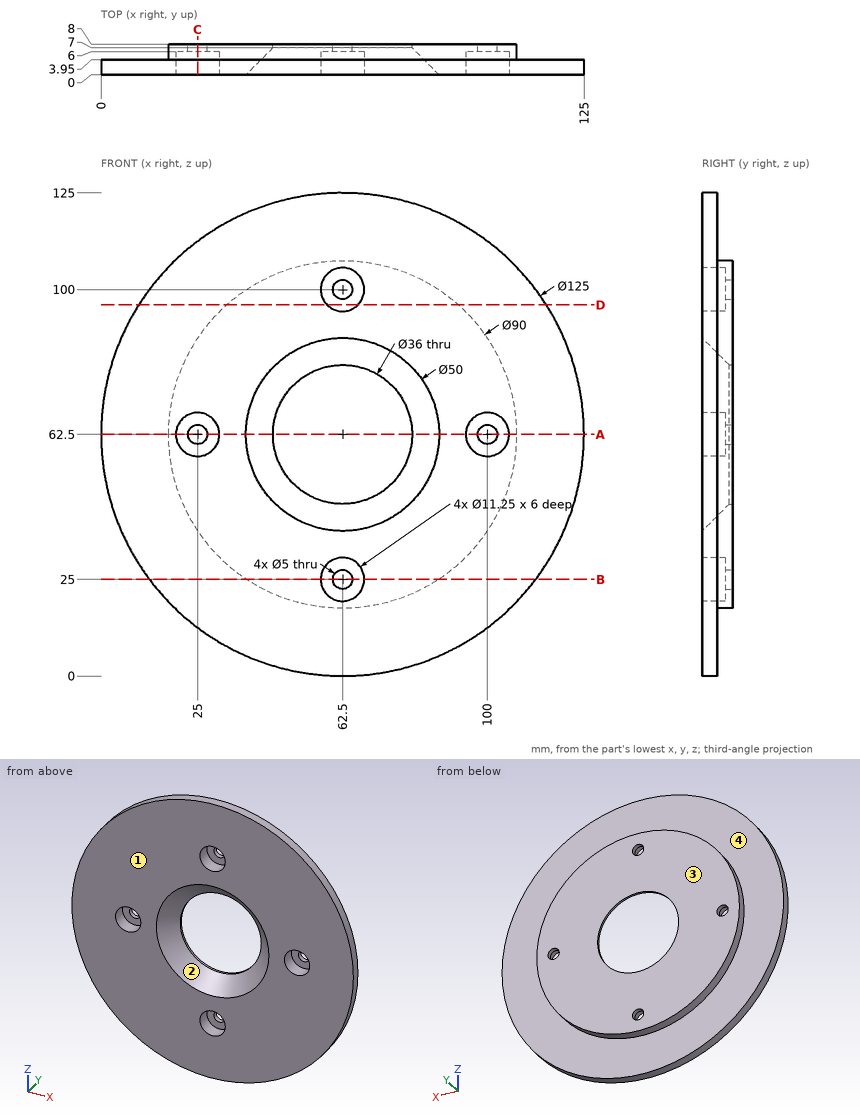
Source: three-view drawing plus pictorial views. Frame: mm from the lowest corner of the part. A direction names the side the tool comes from. Give positions to 0.01 mm unless a question says otherwise; leave off trailing zeros. Order: outer loops, then holes, each group sorted by start corner. A loop starts at its lowest first (then second) coordinate and runs counter-clockwise, first axis right, second up. Notation, with made-up numbers: (-22, -11.75) - (-16, -11.75) arc R23 cw to (-16, 17.25) - close; hole circle Ø6 at (14, -33). An arc over 180 degrees is marked (long way). Answer as a JSON object with one key per item and string values. Group by question number.
Q1. Line query: probe 1 along X at (y, z) = (3, 67.5); probe 2 along Z at (x, y) = (62.5, 7); probe 3 along Z at (x, y) = (62.5, 2.2) (3 decimals). Output: solid intervals per line, ascending.
Q2. Mould query, pull axis X, two halves, no side actions, for the marked faces 1 and 2. Classes: pulls with the +X half, pulls with the -X half, needs draft (parallel to the pull), parting line crosses it, or undercut.
Q3. First-contact query: pin 1 Ø3.5 at (x, z) = (61.5, 101.5) entering from -Y; pin 2 Ø2 at (y, z) = (3.5, 93) entering from +X; pin 3 Ø1 at (x, y) = (61, 1.5) entering from -Z. Flat tips, straight axial feed; report the tip coordinate or a pass-through.
Q4. Cut plane D-D, the plane z = 96. Output: boundary loops of the cut face in (x, y), then the cut area to 3 significant figures.
Q5. Cut plane C-C, the plane x = 25. Output: boundary loops of the cut face in (y, z) (3 decimals), then the cut area to 3 significant figures.
Q6. Cut plane B-B, the plane z = 25. Output: boundary loops of the cut face in (x, y) (3 decimals).
Q7. Set-up query: the marked faces 3 and 4. Return all of +Z, -Z, +X, -X, +Y, -Y with unobstructed straight access to the full face (end or side cutting, diameter ignored); none if empty.
Q8. Cut plane A-A, the plane z = 62.5. Count the separate pieces of the cut face and the enclosed holes in it, then the cut area to 3 significant figures.
Results:
{
 "1": {"probe 1": "0.2 to 22.42, 27.58 to 41.08, 83.92 to 97.42, 102.58 to 124.8", "probe 2": "17.5 to 22.5, 27.5 to 44.5, 80.5 to 97.5, 102.5 to 107.5", "probe 3": "0 to 19.375, 30.625 to 39.7, 85.3 to 94.375, 105.625 to 125"},
 "2": {"face 1": "needs draft", "face 2": "undercut"},
 "3": {"pin 1": "y = 6", "pin 2": "x = 117.6", "pin 3": "z = 0.01"},
 "4": {"outline": "(9.74, 0) - (58.55, 0) - (58.55, 6) - (66.45, 6) - (66.45, 0) - (115.26, 0) - (115.26, 3.95) - (92.55, 3.95) - (92.55, 8) - (32.45, 8) - (32.45, 3.95) - (9.74, 3.95) - close", "area": "613 mm^2"},
 "5": {"outline": "(0, 12.5) - (3.95, 12.5) - (3.95, 37.625) - (8, 37.625) - (8, 60) - (6, 60) - (6, 56.875) - (0, 56.875) - close; (0, 68.125) - (6, 68.125) - (6, 65) - (8, 65) - (8, 87.375) - (3.95, 87.375) - (3.95, 112.5) - (0, 112.5) - close", "area": "519 mm^2"},
 "6": {"outline": "(12.5, 0) - (56.875, 0) - (56.875, 6) - (60, 6) - (60, 8) - (37.625, 8) - (37.625, 3.95) - (12.5, 3.95) - close; (65, 6) - (68.125, 6) - (68.125, 0) - (112.5, 0) - (112.5, 3.95) - (87.375, 3.95) - (87.375, 8) - (65, 8) - close"},
 "7": {"face 3": "+Z, -Z, +X, -X, +Y", "face 4": "+Y"},
 "8": {"separate pieces": "4", "enclosed holes": "0", "area": "366 mm^2"}
}
